Drawing for the job (mm, zero at the part's lowest x, y, z). A direction names the side the tool comes from. Give positions to 0.01 mm unless a question says otherwise; leave off trailing zeros. Order: outer loops, then holes, each group sorted by start corner. A loop starts at its lowest first (then second) coordinate and runs counter-clockwise, first axis right, second up. Notation, with made-up numbers: (51, -3.5) - (84, -3.5) arc R28 ccw to (84, 34.5) - close; hole circle Ø1 at (-28, 54). An arc over 180 degrees is marked (long way). Use a Markdown table: item, result.
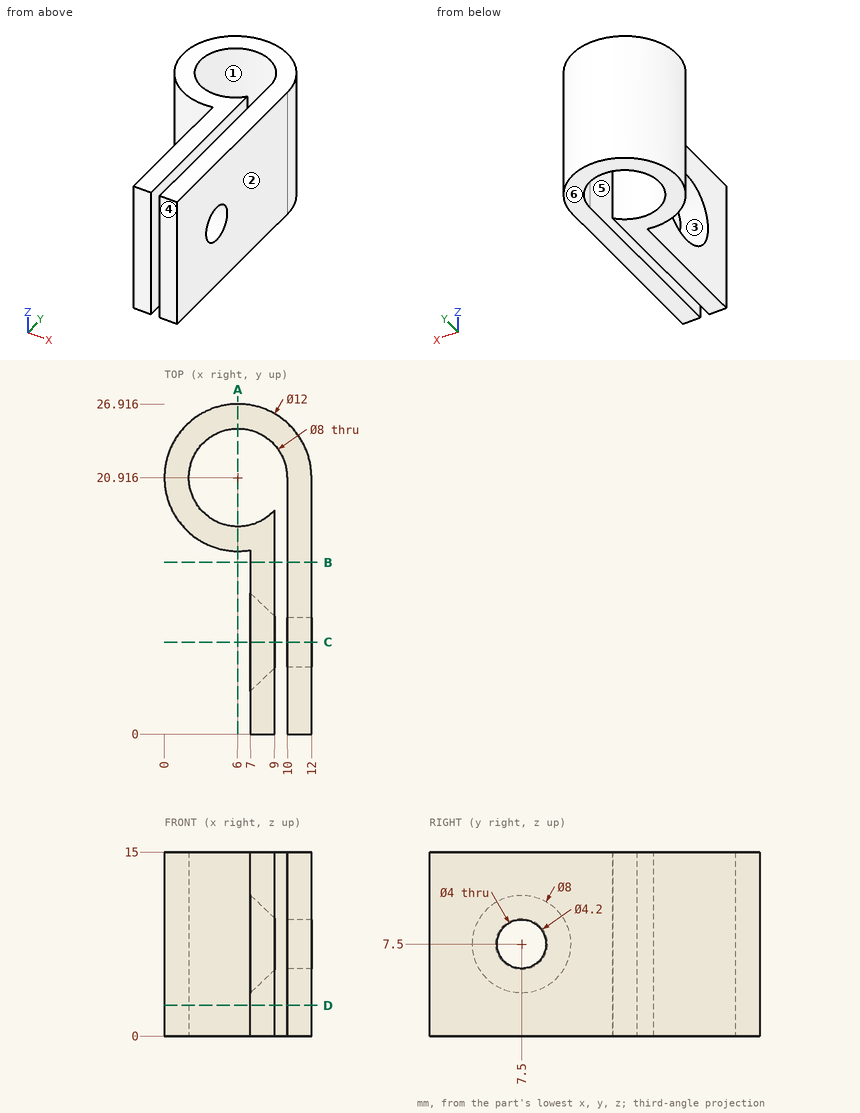
1) Tool access for the marked faces 5 and 6: list every direction of +Z, -Z, +X, -X, +Y, -Y with a clear straight run to the whole face (end or side of a thin tool).
Computed:
| item | result |
|---|---|
| face 5 | +Z, -Z, -Y |
| face 6 | -Z, +X, -X, +Y, -Y |
2) Slice it at B-B (y = 14). Write the cut outline in (x, z).
Computed:
| item | result |
|---|---|
| outline | (7, 0) - (9, 0) - (9, 15) - (7, 15) - close; (10, 0) - (12, 0) - (12, 15) - (10, 15) - close |
3) Slice it at A-A (x = 6). Write the cut outline in (y, z).
Computed:
| item | result |
|---|---|
| outline | (14.92, 0) - (16.92, 0) - (16.92, 15) - (14.92, 15) - close; (24.92, 0) - (26.92, 0) - (26.92, 15) - (24.92, 15) - close |
4) Slice it at D-D (z = 2.5). Write the cut outline in (x, y), and give its area (3 significant figures).
Computed:
| item | result |
|---|---|
| outline | (7, 0) - (9, 0) - (9, 18.27) arc R4 cw (long way) to (10, 20.92) - (10, 0) - (12, 0) - (12, 20.92) arc R6 ccw (long way) to (7, 15) - close |
| area | 126 mm² |
5) Two-plate mould, pull along X, no slides. Class the marked faces 1, 2, 3 and 4: +X half, -X half, draft (parallel to the pull), parting line (faces both ways), or undercut.
Computed:
| item | result |
|---|---|
| face 1 | undercut |
| face 2 | +X half |
| face 3 | -X half |
| face 4 | draft |
6) Wall check: line 1 (X direction, y = 11.5, z = 8.25); line 2 (Y direction, x = 6, z = 11); line 3 (X direction, y = 21, z = 12.5). Give the ranges that are in metal, low to high. Write a range as from..to.
Computed:
| item | result |
|---|---|
| line 1 | x = 7..9, 10..12 |
| line 2 | y = 14.92..16.92, 24.92..26.92 |
| line 3 | x = 0..2, 10..12 |
7) Slice it at C-C (y = 7.5). Write the cut outline in (x, z).
Computed:
| item | result |
|---|---|
| outline | (7, 0) - (9, 0) - (9, 5.4) - (7, 3.5) - close; (7, 11.5) - (9, 9.6) - (9, 15) - (7, 15) - close; (10, 0) - (12, 0) - (12, 5.5) - (10, 5.5) - close; (10, 9.5) - (12, 9.5) - (12, 15) - (10, 15) - close |
8) Pin check, flat tips, straight feed: P1, Ø7.5, axis at y = 13.5, z = 11, coming from the -X side; P2, Ø4, axis at y = 10, z = 9.5, coming from the -X side; P3, Ø1.5, axis at x = 5.5, z = 13, coming from the -Y side. Stop position of each tip, or through.
Computed:
| item | result |
|---|---|
| P1 | stops at x = 1.25 |
| P2 | stops at x = 7 |
| P3 | stops at y = 14.92 |
